Read the model definition and answer for the solid it produces. Units are mm, in the model's axes. Face numbers are marked on the shaded views. A direction names the side the tool comes from. Give positions to 0.01 mm unless a question says otherwise; leave off trailing zeros. Loops run counter-clockwise (first coordinate to the right, second up) from the corner with the lowest first, then second, coordinate; pieces in that order, holes last.
(1) Find section B-B, the plane y = 19.5. Write down the section's boundary in (x, z).
(2) Find section A-A, the plane x = 28. Write down the section's boundary in (y, z), then the cut area to 3 significant figures.
(3) Find section C-C, the plane x = -2. Write down the section's boundary in (y, z).
(4) Find section D-D, the plane y = 9. Write down the section's boundary in (x, z), then the cut area to 3 significant figures.
(5) Which of the six approach directions +Z, -Z, +X, -X, +Y, -Y give full straight-line access (tool end or side, diameter ignored) to the marked faces 1, 2, 3 and 4?
(6) Each of these flat-tipped pins is pushed along its axis until it touches: P1, Ø2.5, axis at y = -9.5, z = 1, coming from the +X side; P2, Ø2, axis at y = 7.5, z = 1.5, coming from the -X side; P3, Ø1, axis at x = 13, z = 1.5, coming from the -Y side. Where does it stop, or does it pass through?
(7) Straight lines are drawn through the part: probe 1 along Y at (x, z) = (18.5, 3.3); probe 2 along X at (y, z) = (24.5, 2); probe 3 along Y at (x, z) = (26, 0.7). For each, find the intervals that lie inside material, in ascending order.
(8) Determine the mould class of the marked faces 5, 6 and 7 for opening direction X: pulls with the +X half, pulls with the -X half, needs draft (parallel to the pull), parting line crosses it, or undercut.
```python
from build123d import *

# Parameters (mm, degrees)
F1_DEPTH = 2
F2_W     = 5
F2_H     = 3
F2_W_2   = 3
F2_H_2   = 5
F3_DEPTH = 3
F4_R     = 3
F5_R     = 2


with BuildPart() as f1:
    # F0 (on Top) → F1 (new body)
    with BuildSketch(Plane.XY):
        Polygon((0, 13.26), (0, 0), (-7.14, 0), (-7.14, -5), (0, -5), (0, -12.14), (5, -12.14), (5, -5), (18.26, -5), (18.26, -12.14), (23.26, -12.14), (23.26, -5), (30.4, -5), (30.4, 0), (23.26, 0), (23.26, 13.26), (30.4, 13.26), (30.4, 18.26), (23.26, 18.26), (23.26, 25.4), (18.26, 25.4), (18.26, 18.26), (5, 18.26), (5, 25.4), (0, 25.4), (0, 18.26), (-7.14, 18.26), (-7.14, 13.26), align=None)
    extrude(amount=F1_DEPTH)

    # F2 (on face) → F3 (join)
    with BuildSketch(Plane.XY.offset(2)):
        with Locations((2.5, 23.9)):
            Rectangle(F2_W, F2_H)
        with Locations((20.76, 23.9)):
            Rectangle(F2_W, F2_H)
        with Locations((-5.64, 15.76)):
            Rectangle(F2_W_2, F2_H_2)
        with Locations((28.9, 15.76)):
            Rectangle(F2_W_2, F2_H_2)
        with Locations((28.9, -2.5)):
            Rectangle(F2_W_2, F2_H_2)
        with Locations((20.76, -10.64)):
            Rectangle(F2_W, F2_H)
        with Locations((2.5, -10.64)):
            Rectangle(F2_W, F2_H)
        with Locations((-5.64, -2.5)):
            Rectangle(F2_W_2, F2_H_2)
    extrude(amount=F3_DEPTH)

    # F4
    f4_edges = [f1.edges().sort_by_distance(p)[0] for p in [
        (18.26, 18.26, 1),
        (5, 18.26, 1),
        (0, 18.26, 1),
        (0, 13.26, 1),
        (0, 0, 1),
        (0, -5, 1),
        (5, -5, 1),
        (18.26, -5, 1),
        (23.26, -5, 1),
        (23.26, 13.26, 1),
        (23.26, 0, 1),
        (23.26, 18.26, 1),
    ]]
    fillet(f4_edges, radius=F4_R)

    # F5
    f5_edges = [f1.edges().sort_by_distance(p)[0] for p in [
        (-5.64, -5, 5),
        (-5.64, 0, 5),
        (-5.64, 13.26, 5),
        (-5.64, 18.26, 5),
        (0, 23.9, 5),
        (5, 23.9, 5),
        (18.26, 23.9, 5),
        (23.26, 23.9, 5),
        (28.9, 13.26, 5),
        (28.9, 18.26, 5),
        (28.9, -5, 5),
        (28.9, 0, 5),
        (23.26, -10.64, 5),
        (18.26, -10.64, 5),
        (5, -10.64, 5),
        (0, -10.64, 5),
    ]]
    fillet(f5_edges, radius=F5_R)


solid = f1.part
```
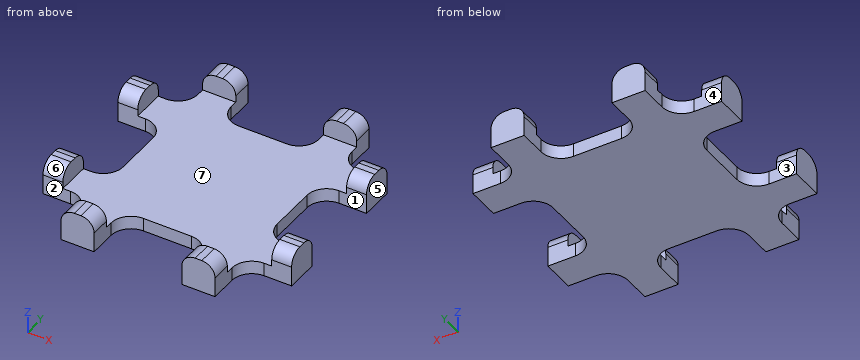
Entries:
1. outline: (-0.57, 0) - (5.57, 0) - (5.57, 2) - (-0.57, 2) - close; (17.69, 0) - (23.83, 0) - (23.83, 2) - (17.69, 2) - close
2. outline: (-5, 0) - (0, 0) - (0, 3) arc R2 ccw to (-2, 5) - (-3, 5) arc R2 ccw to (-5, 3) - close; (13.26, 0) - (18.26, 0) - (18.26, 3) arc R2 ccw to (16.26, 5) - (15.26, 5) arc R2 ccw to (13.26, 3) - close
2. area: 46.6 mm2
3. outline: (-5.17, 0) - (0.17, 0) - (0.17, 2) - (-5.17, 2) - close; (13.09, 0) - (18.43, 0) - (18.43, 2) - (13.09, 2) - close
4. outline: (0, 0) - (23.26, 0) - (23.26, 2) - (0, 2) - close
4. area: 46.5 mm2
5. face 1: +Z, -Z, +X
5. face 2: +Z, -Z, -X, -Y
5. face 3: +Z, -Z, -X
5. face 4: +Z, -Z, -X, +Y
6. P1: stops at x = 23.26
6. P2: stops at x = 0
6. P3: stops at y = -5
7. probe 1: y = -12.14 to -9.14, 22.4 to 25.4
7. probe 2: x = 0 to 5, 18.26 to 23.26
7. probe 3: y = -5.01 to 0.01, 13.25 to 18.27
8. face 5: pulls with the +X half
8. face 6: needs draft
8. face 7: undercut
